```python
from build123d import *

# Parameters (mm, degrees)
PAD_DEPTH       = 30
SKETCH001_W     = 41.77589
SKETCH001_H     = 25.780136
POCKET_DEPTH    = 8.35
SKETCH002_R     = 2.75
POCKET001_DEPTH = 30.001
FILLET_R        = 7
FILLET001_R     = 8
FILLET002_R     = 1
POCKET002_DEPTH = 16.001
CHAMFER_SIZE    = 1
FILLET003_R     = 1


with BuildPart() as part:
    # Sketch → Pad (new body)
    with BuildSketch(Plane.XZ):
        with BuildLine():
            Line((-20, 0), (20, 0))
            Line((20, 10), (20, 0))
            Line((10, 10), (20, 10))
            Line((10, 50), (10, 10))
            ThreePointArc((10, 50), (0, 60), (-10, 50))
            Line((-10, 10), (-10, 50))
            Line((-20, 10), (-10, 10))
            Line((-20, 0), (-20, 10))
        make_face()
    extrude(amount=PAD_DEPTH)

    # Sketch001 (on DatumPlane) → Pocket (cut, symmetric)
    with BuildSketch(Plane(origin=(0, -15, 0), x_dir=(1, 0, 0), z_dir=(0, 1, 0))):
        with Locations((0, -50)):
            Rectangle(SKETCH001_W, SKETCH001_H)
    extrude(amount=POCKET_DEPTH, both=True, mode=Mode.SUBTRACT)

    # Sketch002 (on Face4 of Pocket) → Pocket001 (cut, through all)
    with BuildSketch(Plane(origin=(0, 0, 0), x_dir=(1, 0, 0), z_dir=(0, 1, 0))):
        with Locations((0, -50)):
            Circle(SKETCH002_R)
    extrude(amount=-POCKET001_DEPTH, mode=Mode.SUBTRACT)

    # Fillet
    fillet_edges = [part.edges().sort_by_distance(p)[0] for p in [
        (-10, -15, 37.109932),
        (10, -15, 37.109932),
    ]]
    fillet(fillet_edges, radius=FILLET_R)

    # Fillet001
    fillet001_edges = [part.edges().sort_by_distance(p)[0] for p in [
        (10, -15, 10),
        (-10, -15, 10),
    ]]
    fillet(fillet001_edges, radius=FILLET001_R)

    # Fillet002
    fillet002_edges = [part.edges().sort_by_distance(p)[0] for p in [
        (-20, -15, 10),
        (20, -15, 10),
    ]]
    fillet(fillet002_edges, radius=FILLET002_R)

    # Sketch003 (on DatumPlane) → Pocket002 (cut, through all)
    with BuildSketch(Plane(origin=(0, 0, 16), x_dir=(1, 0, 0), z_dir=(0, 0, -1))):
        with BuildLine():
            ThreePointArc((16.5, 26.507559), (15, 28.007559), (13.5, 26.507559))
            Line((13.5, 26.507559), (13.5, 3.492441))
            ThreePointArc((13.5, 3.492441), (15, 1.992441), (16.5, 3.492441))
            Line((16.5, 26.507559), (16.5, 3.492441))
        make_face()
        with BuildLine():
            ThreePointArc((-13.5, 26.507559), (-15, 28.007559), (-16.5, 26.507559))
            Line((-16.5, 26.507559), (-16.5, 3.49244))
            ThreePointArc((-16.5, 3.49244), (-15, 1.99244), (-13.5, 3.49244))
            Line((-13.5, 26.507559), (-13.5, 3.49244))
        make_face()
    extrude(amount=POCKET002_DEPTH, mode=Mode.SUBTRACT)

    # Chamfer
    chamfer_edges = [part.edges().sort_by_distance(p)[0] for p in [
        (-16.5, -15, 10.141883),
        (-13.5, -15, 11.385622),
        (-14.95623, -1.993079, 10.601658),
        (-14.95623, -28.00692, 10.601658),
        (14.95623, -1.99308, 10.601658),
        (13.5, -15, 11.385622),
        (16.5, -15, 10.141883),
        (14.95623, -28.00692, 10.601658),
    ]]
    chamfer(chamfer_edges, length=CHAMFER_SIZE)

    # Fillet003
    fillet003_edges = [part.edges().sort_by_distance(p)[0] for p in [
        (-10, -23.35, 43.554966),
        (10, -23.35, 43.554966),
        (-10, -6.65, 43.554966),
        (10, -6.65, 43.554966),
    ]]
    fillet(fillet003_edges, radius=FILLET003_R)


solid = part.part
```
The model under review builds one solid part; all positions refer to its coordinate system, in mm. A direction names the side the tool comes from. Coordinates: 2 decimals unless noted, no trailing zeros. Order: outer loops, then holes, each group sorted by start corner. A loop starts at its lowest first (then second) coordinate and runs counter-clockwise, first axis right, second up. Notation, with made-up numbers: M -37.5,68 L -11.5,68 A12 ccw -11.5,73 Z; hole C 50.5,82.5 d6. An arc over 180 degrees is marked long. One line per question, with ' | ' between items.
(1) For probe 1 along Y at (x, z) = (-4, 54.5); probe 2 along Z at (x, y) = (0, -26); probe 3 along X at (y, z) = (-9.5, 19), list the stretches that pass through material, from the lowest coordinate up. Write a range as from..to.
Geometry results:
probe 1: y = -30..-23.35, -6.65..0 | probe 2: z = 0..47.25, 52.75..60 | probe 3: x = -10..10
(2) Insertion check: pin 1 (1 mm diameter, centred on y = -22, z = 33.5, fed in from +X); pin 2 (8 mm diameter, centred on x = 15, y = -4.5, fed in from +Z); pin 3 (1.1 mm diameter, centred on x = -18.5, y = -16.5, fed in from +Z); pin 4 (1.5 mm diameter, centred on x = 11.5, z = 23.5, fed in from +Y). Each pin has a flat end and moves straight along its axis. Give the tip position at first contact, or say it passes through.
Geometry results:
pin 1: stops at x = 9.38 | pin 2: stops at z = 14.13 | pin 3: stops at z = 10 | pin 4: passes through
(3) Add section B-B, the plane x = 0. Write out the cut boundary in (y, z).
Geometry results:
outline: M -30,0 L 0,0 L 0,47.25 L -6.65,47.25 L -6.65,37.11 L -23.35,37.11 L -23.35,47.25 L -30,47.25 Z; M -30,52.75 L -23.35,52.75 L -23.35,59 A1 ccw -24.35,60 L -30,60 Z; M -6.65,52.75 L 0,52.75 L 0,60 L -5.65,60 A1 ccw -6.65,59 Z
(4) The part is to be moulded in two halves that separate along X. For faces 5 (the face through (8.004, -15.131, 35.005)), 6 (the face through (0, -27, 60)), 7 (the face through (13.5, -15, 5)), say which applies: +X half, -X half, draft (parallel to the pull), parting line (faces both ways), or undercut.
Geometry results:
face 5: +X half | face 6: parting line | face 7: undercut
(5) Add section A-A, the plane y = -14. Write out the cut boundary in (x, z), then the cut area to 3 significant figures.
Geometry results:
outline: M -20,0 L -16.5,0 L -16.5,9.14 L -17.49,10.02 A8 cw -18,10 L -19,10 A1 ccw -20,9 Z; M -13.5,0 L 13.5,0 L 13.5,10.39 L 12.71,12 A8 cw 10,18 L 10,30.11 A7 ccw 3,37.11 L -3,37.11 A7 ccw -10,30.11 L -10,18 A8 cw -12.71,12 L -13.5,10.39 Z; M 16.5,0 L 20,0 L 20,9 A1 ccw 19,10 L 18,10 A8 cw 17.49,10.02 L 16.5,9.14 Z | area: 883 mm²
(6) Add section C-C, the plane z = 21.5. Write out the cut boundary in (x, y).
Geometry results:
outline: M -10,-30 L 10,-30 L 10,0 L -10,0 Z
(7) Add section D-D, the plane z = 32. Write out the cut boundary in (x, y).
Geometry results:
outline: M -10,-30 L 10,-30 L 10,-24.35 A1 ccw 9.74,-23.68 L 9.74,-6.32 A1 ccw 10,-5.65 L 10,0 L -10,0 L -10,-5.65 A1 ccw -9.74,-6.32 L -9.74,-23.68 A1 ccw -10,-24.35 Z
(8) Machinability: for faces 1 (the face through (-14.967, -28.007, 5.266)), 2 (the face through (10, -15, 27)), 3 (the face through (0, -15, 37.11)), 4 (the face through (-10, -15, 27)), which of the approach directions +Z, -Z, +X, -X, +Y, -Y give a long, thin tool a straight path to every point of the face, cutting with its end or side? Answer none if there is none.
Geometry results:
face 1: +Z, -Z | face 2: +Z, +X, +Y, -Y | face 3: +Z, +X, -X | face 4: +Z, -X, +Y, -Y
